Autodesk Inventor part; units mm, degrees
ref_plane "YZ Plane" through (0, 0, 0) normal (1, 0, 0) x (0, 1, 0)
ref_plane "XZ Plane" through (0, 0, 0) normal (0, 1, 0) x (-1, 0, 0)
ref_plane "XY Plane" through (0, 0, 0) normal (0, 0, 1) x (1, 0, 0)
sketch "Sketch1" plane through (0, 0, 0) normal (0, 1, 0) x (-1, 0, 0)
  circle A0 centre (0, 0) radius 1.5
  dimension "d0" = 3
extrude "Extrusion1" add sketch "Sketch1" along normal blind 6
sketch "Sketch2" plane through (0, 6, 0) normal (0, 1, 0) x (1, 0, 0)
  circle A0 centre (0, 0) radius 2.5
  dimension "d3" = 5
extrude "Extrusion2" add sketch "Sketch2" along normal blind 2
fillet "Fillet1" radius 1.7 1 edges at (-2.5, 8, 0)
chamfer "Chamfer1" distance 0.3 angle 45 1 edges at (1.5, 0, 0)
thread "Thread1"
properties part number "M3x6 Screw Nylon" material "Nylon 6"
Source: CAD feature listing. Evaluate the final solid. Frame: model axes, mm. A direction names the side the tool comes from. Round coordinates to 2 decimals unless told otherwise and drop trailing zeros. Loops run counter-clockwise (first coordinate to the right, second up) from the corner with the lowest first, then second, coordinate; pieces in that order, holes last. Notation, with made-up numbers: M -28,59.5 L -17,59.5 A31 cw -17,93.5 Z; hole C 46,66 d5. An arc over 180 degrees is marked long. Use a Markdown table: item, result. Add a question column.
1. Reachability of faces 1 (the flat face through (0, 8, 0)), 2 (the cylindrical face through (1.5, 3.11, -0.07)) from +Z, -Z, +X, -X, +Y, -Y: full face, straight path, thin tool, end or side. Return the list, or none.
2. Contact query for flat-ended pins moving along their axis: P1, Ø3, axis at y = 4, z = 0, coming from the -X side; P2, Ø1.5, axis at x = 2, y = 3.5, coming from the +Z side; P3, Ø1.5, axis at x = 0, z = 1, coming from the -Y side; P4, Ø1.5, axis at x = 0, y = 2, coming from the +Z side. Output: stop coordinate, or through.
3. Section query A-A on y = 0.5. Return the cut outline in (x, z), then the cut area to 3 significant figures.
4. Line query: line 1 (Z direction, x = 0.9, y = 5); line 2 (Y direction, x = -0.3, z = 1.7); line 3 (Y direction, x = 1.65, z = -1.55). Output: solid intervals per line, ascending.
Reported:
| question | item | result |
|---|---|---|
| 1 | face 1 | +Z, -Z, +X, -X, +Y |
| 1 | face 2 | -Y |
| 2 | P1 | stops at x = -1.5 |
| 2 | P2 | stops at z = 0.83 |
| 2 | P3 | stops at y = 0 |
| 2 | P4 | stops at z = 1.5 |
| 3 | outline | C 0,0 d3 |
| 3 | area | 7.07 mm² |
| 4 | line 1 | z = -1.2 to 1.2 |
| 4 | line 2 | y = 6 to 7.73 |
| 4 | line 3 | y = 6 to 7.16 |
